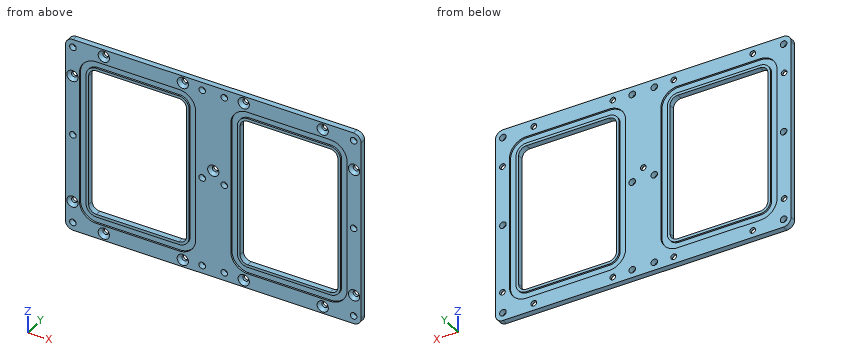
```python
from build123d import *

# Parameters (mm, degrees)
F1_DEPTH       = 3.302
F3_DEPTH       = 1.016
F6_D           = 3.2639
F6_CSINK_D     = 6.477
F6_CSINK_ANGLE = 82
F8_D           = 3.7973


# Not quite as in the source:
# - a pattern or mirror of a feature is missing from the dataset's text; its kind, count and spacing are read off the source's solid


with BuildPart() as f1:
    # F0 (on Front) → F1 (new body)
    with BuildSketch(Plane.XZ):
        with BuildLine():
            ThreePointArc((-85.09, -51.7525), (-83.7880896424, -54.8955896424), (-80.645, -56.1975))
            Line((-80.645, -56.1975), (80.645, -56.1975))
            ThreePointArc((80.645, -56.1975), (83.7880896424, -54.8955896424), (85.09, -51.7525))
            Line((85.09, -51.7525), (85.09, 51.7525))
            ThreePointArc((85.09, 51.7525), (83.7880896424, 54.8955896424), (80.645, 56.1975))
            Line((80.645, 56.1975), (-80.645, 56.1975))
            ThreePointArc((-80.645, 56.1975), (-83.7880896424, 54.8955896424), (-85.09, 51.7525))
            Line((-85.09, 51.7525), (-85.09, -51.7525))
        make_face()
        with BuildLine():
            ThreePointArc((-15.4305, -37.846), (-16.7324103576, -40.9890896424), (-19.8755, -42.291))
            Line((-19.8755, -42.291), (-67.2465, -42.291))
            ThreePointArc((-67.2465, -42.291), (-70.3895896424, -40.9890896424), (-71.6915, -37.846))
            Line((-71.6915, -37.846), (-71.6915, 37.846))
            ThreePointArc((-71.6915, 37.846), (-70.3895896424, 40.9890896424), (-67.2465, 42.291))
            Line((-67.2465, 42.291), (-19.8755, 42.291))
            ThreePointArc((-19.8755, 42.291), (-16.7324103576, 40.9890896424), (-15.4305, 37.846))
            Line((-15.4305, 37.846), (-15.4305, -37.846))
        make_face(mode=Mode.SUBTRACT)
        with BuildLine():
            Line((19.8755, 42.291), (67.2465, 42.291))
            ThreePointArc((67.2465, 42.291), (70.3895896424, 40.9890896424), (71.6915, 37.846))
            Line((71.6915, 37.846), (71.6915, -37.846))
            ThreePointArc((71.6915, -37.846), (70.3895896424, -40.9890896424), (67.2465, -42.291))
            Line((67.2465, -42.291), (19.8755, -42.291))
            ThreePointArc((19.8755, -42.291), (16.7324103576, -40.9890896424), (15.4305, -37.846))
            Line((15.4305, -37.846), (15.4305, 37.846))
            ThreePointArc((15.4305, 37.846), (16.7324103576, 40.9890896424), (19.8755, 42.291))
        make_face(mode=Mode.SUBTRACT)
    extrude(amount=F1_DEPTH)

    # F2 (on face) → F3 (cut)
    with BuildSketch(Plane.XZ.offset(3.302)):
        with BuildLine():
            ThreePointArc((-10.0965, 37.846), (-12.9607027868, 44.7607972132), (-19.8755, 47.625))
            Line((-19.8755, 47.625), (-67.2465, 47.625))
            ThreePointArc((-67.2465, 47.625), (-74.1612972132, 44.7607972132), (-77.0255, 37.846))
            Line((-77.0255, 37.846), (-77.0255, -37.846))
            ThreePointArc((-77.0255, -37.846), (-74.1612972132, -44.7607972132), (-67.2465, -47.625))
            Line((-67.2465, -47.625), (-19.8755, -47.625))
            ThreePointArc((-19.8755, -47.625), (-12.9607027868, -44.7607972132), (-10.0965, -37.846))
            Line((-10.0965, -37.846), (-10.0965, 37.846))
        make_face()
        with BuildLine():
            ThreePointArc((-19.8755, 43.815), (-15.6547796231, 42.0667203769), (-13.9065, 37.846))
            Line((-13.9065, 37.846), (-13.9065, -37.846))
            ThreePointArc((-13.9065, -37.846), (-15.6547796231, -42.0667203769), (-19.8755, -43.815))
            Line((-19.8755, -43.815), (-67.2465, -43.815))
            ThreePointArc((-67.2465, -43.815), (-71.4672203769, -42.0667203769), (-73.2155, -37.846))
            Line((-73.2155, -37.846), (-73.2155, 37.846))
            ThreePointArc((-73.2155, 37.846), (-71.4672203769, 42.0667203769), (-67.2465, 43.815))
            Line((-67.2465, 43.815), (-19.8755, 43.815))
        make_face(mode=Mode.SUBTRACT)
        with BuildLine():
            ThreePointArc((10.0965, -37.846), (12.9607027868, -44.7607972132), (19.8755, -47.625))
            Line((19.8755, -47.625), (67.2465, -47.625))
            ThreePointArc((67.2465, -47.625), (74.1612972132, -44.7607972132), (77.0255, -37.846))
            Line((77.0255, -37.846), (77.0255, 37.846))
            ThreePointArc((77.0255, 37.846), (74.1612972132, 44.7607972132), (67.2465, 47.625))
            Line((67.2465, 47.625), (19.8755, 47.625))
            ThreePointArc((19.8755, 47.625), (12.9607027868, 44.7607972132), (10.0965, 37.846))
            Line((10.0965, 37.846), (10.0965, -37.846))
        make_face()
        with BuildLine():
            Line((73.2155, 37.846), (73.2155, -37.846))
            ThreePointArc((73.2155, -37.846), (71.4672203769, -42.0667203769), (67.2465, -43.815))
            Line((67.2465, -43.815), (19.8755, -43.815))
            ThreePointArc((19.8755, -43.815), (15.6547796231, -42.0667203769), (13.9065, -37.846))
            Line((13.9065, -37.846), (13.9065, 37.846))
            ThreePointArc((13.9065, 37.846), (15.6547796231, 42.0667203769), (19.8755, 43.815))
            Line((19.8755, 43.815), (67.2465, 43.815))
            ThreePointArc((67.2465, 43.815), (71.4672203769, 42.0667203769), (73.2155, 37.846))
        make_face(mode=Mode.SUBTRACT)
    f3 = extrude(amount=-F3_DEPTH, mode=Mode.SUBTRACT)

    # F3_copies: F3 across plane
    add(f3.mirror(Plane.ZX.offset(-1.651)), mode=Mode.SUBTRACT)

    # F6 (through all)
    with Locations(Plane.XZ.offset(3.302)):
        with Locations((-81.026, 34.6075), (-81.026, -39.4335), (-62.992, 52.1335), (-17.526, 52.1335), (0, 6.4135), (-62.992, -52.1335), (-17.526, -52.1335), (17.526, -52.1335), (62.992, -52.1335), (81.026, -39.4335), (81.026, 34.6075), (62.992, 52.1335), (17.526, 52.1335)):
            CounterSinkHole(F6_D / 2, F6_CSINK_D / 2, counter_sink_angle=F6_CSINK_ANGLE)

    # F8 (through all)
    with Locations(Plane.XZ.offset(3.302)):
        with Locations((-80.772, 51.6255), (-80.772, 0), (-80.772, -51.6255), (-6.35, -51.6255), (-6.35, 0), (6.35, 0), (-6.35, 51.6255), (6.35, 51.6255), (6.35, -51.6255), (80.772, -51.6255), (80.772, 51.6255), (80.772, 0)):
            Hole(F8_D / 2)


solid = f1.part
```
Read the model definition and answer for the solid it produces. Units are mm, in the model's axes. Give positions to 0.01 mm unless a question says otherwise; leave off trailing zeros. Order: outer loops, then holes, each group sorted by start corner. A loop starts at its lowest first (then second) coordinate and runs counter-clockwise, first axis right, second up. Notation, with made-up numbers: (-30.5, 33) -> (-26.5, 33) arc R17 ccw to (-26.5, 56) -> close; hole circle Ø1 at (75, 88). An arc over 180 degrees is marked (long way). One line per item, written item: value. Start each with the question number.
(1) The part is cut by section B-B (z = 0). State how many separate pieces and enclosed holes the cut face has, and give its area (3 significant figures).
(2) Flat-ended cylindrical pins translate along their axes: P1, Ø1, axis at x = 9, z = 25, coming from the +Y side; P2, Ø4, axis at x = -17.53, z = 52.13, coming from the -Y side. Find the tip coordinate at first contact, or state that the pin passes through.
(3) The part is cut by section C-C (x = 23). Determine the outline of the cut face in (y, z) (1 decimal).
(4) Straight lines are drawn through the part: L1, parallel to X at y = -1.35, z = 18; L2, parallel to Z at x = 43.5, y = -0.3 (1 decimal); L3, parallel to Z at x = 42, y = -1.25. For each, find the intervals that lie inside material, in ascending order.
(5) The part is cut by section A-A (x = 0). Determine the outline of the cut face in (y, z) (1 decimal).
Taken from the geometry:
1. separate pieces: 7
1. enclosed holes: 0
1. area: 109 mm^2
2. P1: y = 0
2. P2: y = -1.88
3. outline: (-3.3, -56.2) -> (0, -56.2) -> (0, -47.6) -> (-1, -47.6) -> (-1, -43.8) -> (0, -43.8) -> (0, -42.3) -> (-3.3, -42.3) -> (-3.3, -43.8) -> (-2.3, -43.8) -> (-2.3, -47.6) -> (-3.3, -47.6) -> close; (-3.3, 42.3) -> (0, 42.3) -> (0, 43.8) -> (-1, 43.8) -> (-1, 47.6) -> (0, 47.6) -> (0, 56.2) -> (-3.3, 56.2) -> (-3.3, 47.6) -> (-2.3, 47.6) -> (-2.3, 43.8) -> (-3.3, 43.8) -> close
4. L1: -85.09 to -71.69, -15.43 to 15.43, 71.69 to 85.09
4. L2: -56.2 to -47.6, -43.8 to -42.3, 42.3 to 43.8, 47.6 to 56.2
4. L3: -56.2 to -42.29, 42.29 to 56.2
5. outline: (-3.3, -56.2) -> (0, -56.2) -> (0, 4.8) -> (-1.5, 4.8) -> (-3.3, 3.2) -> close; (-3.3, 9.7) -> (-1.5, 8) -> (0, 8) -> (0, 56.2) -> (-3.3, 56.2) -> close
